For this review, take the finished solid that the model builds, in its own axes (mm). Face numbers are marked on the shaded views. A direction names the side the tool comes from. Give positions to 0.01 mm unless a question says otherwise; leave off trailing zeros. Write each loop counter-clockwise with the first axis right and the second up, starting at its lowest first coordinate (ties: lowest second). Pieces come first, ordered by that corner, then holes. Notation, with made-up numbers: (24.5, 62) -> (76.5, 62) arc R32 ccw to (76.5, 93) -> close; hole circle Ø7 at (-35, -0.75). An arc over 180 degrees is marked (long way). Return JSON: item names as keys, results as strings.
from build123d import *

# Parameters (mm, degrees)
BOSS_EXTRUDE1_DEPTH = 28
SKETCH3_R           = 5.75
SKETCH3_R_2         = 1.3
CUT_EXTRUDE1_DEPTH  = 79.74007874
SKETCH4_R           = 1.7
CUT_EXTRUDE2_DEPTH  = 25
FILLET1_R           = 2
FILLET2_R           = 12.5
CUT_EXTRUDE3_DEPTH  = 2.5
SKETCH6_R           = 2.75
CUT_EXTRUDE4_DEPTH  = 2
CUT_EXTRUDE5_START  = -2
SKETCH9_R           = 2.75
CUT_EXTRUDE5_DEPTH  = 2


with BuildPart() as part:
    # Sketch1 → Boss-Extrude1 (new body)
    with BuildSketch(Plane(origin=(0, 0, 0), x_dir=(1, 0, 0), z_dir=(0, 1, 0))):
        Polygon((-27, 50), (-27, -4.5), (27, -4.5), (27, 50), (23.5, 50), (23.5, 0), (-23.5, 0), (-23.5, 50), align=None)
    extrude(amount=BOSS_EXTRUDE1_DEPTH)

    # Sketch3 → Cut-Extrude1 (cut, through all)
    with BuildSketch(Plane(origin=(27, 0, 0), x_dir=(0, 0, -1), z_dir=(1, 0, 0))):
        with Locations((35, 14)):
            Circle(SKETCH3_R)
        with Locations((46, 14)):
            Circle(SKETCH3_R_2)
        with Locations((35, 3)):
            Circle(SKETCH3_R_2)
        with Locations((24, 14)):
            Circle(SKETCH3_R_2)
        with Locations((35, 25)):
            Circle(SKETCH3_R_2)
    extrude(amount=-CUT_EXTRUDE1_DEPTH, mode=Mode.SUBTRACT)

    # Sketch4 → Cut-Extrude2 (cut)
    with BuildSketch(Plane.XY.offset(4.5)):
        with Locations((-17.5, 6.5)):
            Circle(SKETCH4_R)
        with Locations((17.5, 6.5)):
            Circle(SKETCH4_R)
        with Locations((17.5, 21.5)):
            Circle(SKETCH4_R)
        with Locations((-17.5, 21.5)):
            Circle(SKETCH4_R)
    extrude(amount=-CUT_EXTRUDE2_DEPTH, mode=Mode.SUBTRACT)

    # Fillet1
    fillet1_edges = [part.edges().sort_by_distance(p)[0] for p in [
        (-23.5, 14, 0),
        (23.5, 14, 0),
        (27, 14, 4.5),
        (-27, 14, 4.5),
    ]]
    fillet(fillet1_edges, radius=FILLET1_R)

    # Fillet2
    fillet2_edges = [part.edges().sort_by_distance(p)[0] for p in [
        (-25.25, 0, -50),
        (25.25, 28, -50),
        (-25.25, 28, -50),
        (25.25, 0, -50),
    ]]
    fillet(fillet2_edges, radius=FILLET2_R)

    # Sketch5 → Cut-Extrude3 (cut)
    with BuildSketch(Plane(origin=(0, 0, 0), x_dir=(-1, 0, 0), z_dir=(0, 0, -1))):
        Polygon((19.174315781, 18.6), (20.848631561, 21.5), (19.174315781, 24.4), (15.825684219, 24.4), (14.151368439, 21.5), (15.825684219, 18.6), align=None)
        Polygon((-15.825684219, 18.6), (-14.151368439, 21.5), (-15.825684219, 24.4), (-19.174315781, 24.4), (-20.848631561, 21.5), (-19.174315781, 18.6), align=None)
        Polygon((19.174315781, 3.6), (20.848631561, 6.5), (19.174315781, 9.4), (15.825684219, 9.4), (14.151368439, 6.5), (15.825684219, 3.6), align=None)
        Polygon((-15.825684219, 3.6), (-14.151368439, 6.5), (-15.825684219, 9.4), (-19.174315781, 9.4), (-20.848631561, 6.5), (-19.174315781, 3.6), align=None)
    extrude(amount=-CUT_EXTRUDE3_DEPTH, mode=Mode.SUBTRACT)

    # Sketch6 → Cut-Extrude4 (cut)
    with BuildSketch(Plane(origin=(27, 0, 0), x_dir=(0, 0, -1), z_dir=(1, 0, 0))):
        with Locations((24, 14)):
            Circle(SKETCH6_R)
        with Locations((35, 25)):
            Circle(SKETCH6_R)
        with Locations((46, 14)):
            Circle(SKETCH6_R)
        with Locations((35, 3)):
            Circle(SKETCH6_R)
    extrude(amount=-CUT_EXTRUDE4_DEPTH, mode=Mode.SUBTRACT)

    # Sketch9 → Cut-Extrude5 (cut)
    with BuildSketch(Plane.ZY.offset(27).offset(CUT_EXTRUDE5_START)):
        with Locations(Location((-46, 14, 0), (0, 0, 180))):
            Circle(SKETCH9_R)
        with Locations(Location((-35, 25, 0), (0, 0, 180))):
            Circle(SKETCH9_R)
        with Locations(Location((-24, 14, 0), (0, 0, 180))):
            Circle(SKETCH9_R)
        with Locations(Location((-35, 3, 0), (0, 0, 180))):
            Circle(SKETCH9_R)
    extrude(amount=CUT_EXTRUDE5_DEPTH, mode=Mode.SUBTRACT)


solid = part.part
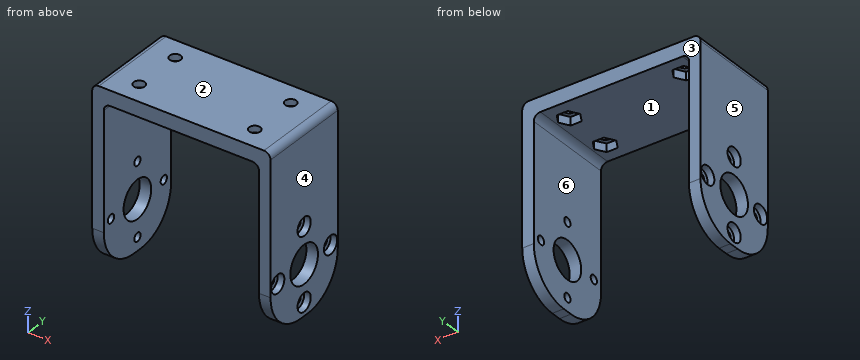
1. The part is to be moulded in two halves that separate along X. For the marked faces 3, 4, 5 and 6, say which applies: +X half, -X half, draft (parallel to the pull), parting line (faces both ways), or undercut.
Results found:
{"face 3": "draft", "face 4": "+X half", "face 5": "-X half", "face 6": "undercut"}
2. Add section B-B, the plane z = -15. State the section outline as (x, y) points, plus the area to 3 significant figures.
Results found:
{"outline": "(-27, 0) -> (-23.5, 0) -> (-23.5, 28) -> (-27, 28) -> close; (23.5, 0) -> (27, 0) -> (27, 28) -> (23.5, 28) -> close", "area": "196 mm²"}
3. For the marked faces 1 and 2, list the 3-axis set-ups (+Z, -Z, +X, -X, +Y, -Y) from which the entire face can be reached by the end or side of a thin tool; tool diameter is ignored.
Results found:
{"face 1": "-Z, +Y, -Y", "face 2": "+Z, +X, -X, +Y, -Y"}
4. To check wall thickness, follow probe 1 along Y at (x, z) = (-26.25, -35); probe 2 along X at (y, z) = (22.75, -37); probe 3 along Y at (x, z) = (-17, 3). State the ranges of each line that lie inside material, in increasing order.
Results found:
{"probe 1": "y = 0 to 0.25, 5.75 to 8.25, 19.75 to 22.25, 27.75 to 28", "probe 2": "x = -27 to -23.5, 23.5 to 27", "probe 3": "y = 0 to 4.88, 8.12 to 19.88, 23.12 to 28"}
5. Add section C-C, the plane z = -46. State the section outline as (x, y) points.
Results found:
{"outline": "(-27, 3.33) -> (-23.5, 3.33) -> (-23.5, 12.7) -> (-25, 12.7) -> (-25, 11.25) -> (-27, 11.25) -> close; (-27, 16.75) -> (-25, 16.75) -> (-25, 15.3) -> (-23.5, 15.3) -> (-23.5, 24.67) -> (-27, 24.67) -> close; (23.5, 3.33) -> (27, 3.33) -> (27, 11.25) -> (25, 11.25) -> (25, 12.7) -> (23.5, 12.7) -> close; (23.5, 15.3) -> (25, 15.3) -> (25, 16.75) -> (27, 16.75) -> (27, 24.67) -> (23.5, 24.67) -> close"}
6. Add section A-A, the plane x = -17.5. State the section outline as (y, z) points.
Results found:
{"outline": "(0, 0) -> (3.6, 0) -> (3.6, 2.5) -> (4.8, 2.5) -> (4.8, 4.5) -> (0, 4.5) -> close; (8.2, 2.5) -> (9.4, 2.5) -> (9.4, 0) -> (18.6, 0) -> (18.6, 2.5) -> (19.8, 2.5) -> (19.8, 4.5) -> (8.2, 4.5) -> close; (23.2, 2.5) -> (24.4, 2.5) -> (24.4, 0) -> (28, 0) -> (28, 4.5) -> (23.2, 4.5) -> close"}
7. For pin 1 (4 mm diameter, centred on x = 1.5, y = 13.5, fed in from -Z); pin 2 (4.5 mm diameter, centred on x = -17.5, y = 21.5, fed in from -Z); pin 3 (4.5 mm diameter, centred on y = 25, z = -35, fed in from +X), all flat-tipped, find the tip position at first contact; note any pin that passes through.
Results found:
{"pin 1": "stops at z = 0", "pin 2": "stops at z = 2.5", "pin 3": "stops at x = 25"}
8. Add section D-D, the plane y = 7.5. State the section outline as (x, z) points.
Results found:
{"outline": "(-27, -48.96) -> (-23.5, -48.96) -> (-23.5, -2) arc R2 cw to (-21.5, 0) -> (-20.27, 0) -> (-20.27, 2.5) -> (-18.87, 2.5) -> (-18.87, 4.5) -> (-25, 4.5) arc R2 ccw to (-27, 2.5) -> close; (-16.13, 2.5) -> (-14.73, 2.5) -> (-14.73, 0) -> (14.73, 0) -> (14.73, 2.5) -> (16.13, 2.5) -> (16.13, 4.5) -> (-16.13, 4.5) -> close; (18.87, 2.5) -> (20.27, 2.5) -> (20.27, 0) -> (21.5, 0) arc R2 cw to (23.5, -2) -> (23.5, -48.96) -> (27, -48.96) -> (27, 2.5) arc R2 ccw to (25, 4.5) -> (18.87, 4.5) -> close"}
